from build123d import *

# Parameters (mm, degrees)
SKETCH1_R           = 0.5
SKETCH1_R_2         = 1.375
BOSS_EXTRUDE1_DEPTH = 2
SKETCH4_R           = 4.5
SKETCH4_R_2         = 2.5
BOSS_EXTRUDE3_DEPTH = 3
CUT_EXTRUDE3_START  = -3
CUT_EXTRUDE3_DEPTH  = 3
SKETCH6_W           = 34.029642768
SKETCH6_H           = 33.796563024
CUT_EXTRUDE4_DEPTH  = 22.43595111
SKETCH7_W           = 10.1
SKETCH7_H           = 10.1
BOSS_EXTRUDE4_DEPTH = 1.25
SKETCH8_W           = 1.25
SKETCH8_H           = 10.1
BOSS_EXTRUDE5_DEPTH = 2


with BuildPart() as part:
    # Sketch1 → Boss-Extrude1 (new body)
    with BuildSketch(Plane(origin=(0, 0, 0), x_dir=(1, 0, 0), z_dir=(0, 1, 0))):
        with BuildLine():
            Line((-4, 4), (-2.467435953, 13.402193757))
            ThreePointArc((-2.467435953, 13.402193757), (0, 15.5), (2.467435953, 13.402193757))
            Line((2.467435953, 13.402193757), (4, 4))
            Line((4, 4), (12.448472752, 2.459445505))
            ThreePointArc((12.448472752, 2.459445505), (14.5, 0), (12.448472752, -2.459445505))
            Line((12.448472752, -2.459445505), (4, -4))
            Line((4, -4), (2.467435953, -13.402193757))
            ThreePointArc((2.467435953, -13.402193757), (0, -15.5), (-2.467435953, -13.402193757))
            Line((-2.467435953, -13.402193757), (-4, -4))
            Line((-4, -4), (-12.448472752, -2.459445505))
            ThreePointArc((-12.448472752, -2.459445505), (-14.5, 0), (-12.448472752, 2.459445505))
            Line((-12.448472752, 2.459445505), (-4, 4))
        make_face()
        with Locations(Location((0, 12, 0), (0, 0, 270))):
            Circle(SKETCH1_R, mode=Mode.SUBTRACT)
        with Locations(Location((0, 9.5, 0), (0, 0, 270))):
            Circle(SKETCH1_R, mode=Mode.SUBTRACT)
        with Locations(Location((0, 7.5, 0), (0, 0, 270))):
            Circle(SKETCH1_R, mode=Mode.SUBTRACT)
        with Locations(Location((12, 0, 0), (0, 0, 270))):
            Circle(SKETCH1_R, mode=Mode.SUBTRACT)
        with Locations(Location((9.5, 0, 0), (0, 0, 270))):
            Circle(SKETCH1_R, mode=Mode.SUBTRACT)
        with Locations(Location((7.5, 0, 0), (0, 0, 270))):
            Circle(SKETCH1_R, mode=Mode.SUBTRACT)
        with Locations(Location((0, -12, 0), (0, 0, 270))):
            Circle(SKETCH1_R, mode=Mode.SUBTRACT)
        with Locations(Location((0, -9.5, 0), (0, 0, 270))):
            Circle(SKETCH1_R, mode=Mode.SUBTRACT)
        with Locations(Location((0, -7.5, 0), (0, 0, 270))):
            Circle(SKETCH1_R, mode=Mode.SUBTRACT)
        with Locations(Location((-12, 0, 0), (0, 0, 270))):
            Circle(SKETCH1_R, mode=Mode.SUBTRACT)
        with Locations(Location((-9.5, 0, 0), (0, 0, 270))):
            Circle(SKETCH1_R, mode=Mode.SUBTRACT)
        with Locations(Location((-7.5, 0, 0), (0, 0, 270))):
            Circle(SKETCH1_R, mode=Mode.SUBTRACT)
        with Locations(Location((0, 0, 0), (0, 0, 270))):
            Circle(SKETCH1_R_2, mode=Mode.SUBTRACT)
    extrude(amount=BOSS_EXTRUDE1_DEPTH)

    # Sketch4 → Boss-Extrude3 (add)
    with BuildSketch(Plane.XZ):
        with Locations(Location((0, 0, 0), (0, 0, 90))):
            Circle(SKETCH4_R)
        with Locations(Location((0, 0, 0), (0, 0, 270))):
            Circle(SKETCH4_R_2, mode=Mode.SUBTRACT)
    extrude(amount=BOSS_EXTRUDE3_DEPTH)

    # Sketch5 → Cut-Extrude3 (cut)
    with BuildSketch(Plane.XZ.offset(3).offset(CUT_EXTRUDE3_START)):
        with BuildLine():
            Line((0.299038106, 2.482050808), (0, 3))
            Line((0, 3), (-0.299038106, 2.482050808))
            ThreePointArc((-0.299038106, 2.482050808), (-0.391086163, 2.469220851), (-0.482593741, 2.452978451))
            Line((-0.482593741, 2.452978451), (-0.927050983, 2.853169549))
            Line((-0.927050983, 2.853169549), (-1.051398019, 2.268162738))
            ThreePointArc((-1.051398019, 2.268162738), (-1.134976249, 2.22751631), (-1.216985951, 2.183791473))
            Line((-1.216985951, 2.183791473), (-1.763355757, 2.427050983))
            Line((-1.763355757, 2.427050983), (-1.70083977, 1.832251096))
            ThreePointArc((-1.70083977, 1.832251096), (-1.767766953, 1.767766953), (-1.832251096, 1.70083977))
            Line((-1.832251096, 1.70083977), (-2.427050983, 1.763355757))
            Line((-2.427050983, 1.763355757), (-2.183791473, 1.216985951))
            ThreePointArc((-2.183791473, 1.216985951), (-2.22751631, 1.134976249), (-2.268162738, 1.051398019))
            Line((-2.268162738, 1.051398019), (-2.853169549, 0.927050983))
            Line((-2.853169549, 0.927050983), (-2.452978451, 0.482593741))
            ThreePointArc((-2.452978451, 0.482593741), (-2.469220851, 0.391086163), (-2.482050808, 0.299038106))
            Line((-2.482050808, 0.299038106), (-3, 0))
            Line((-3, 0), (-2.482050808, -0.299038106))
            ThreePointArc((-2.482050808, -0.299038106), (-2.469220851, -0.391086163), (-2.452978451, -0.482593741))
            Line((-2.452978451, -0.482593741), (-2.853169549, -0.927050983))
            Line((-2.853169549, -0.927050983), (-2.268162738, -1.051398019))
            ThreePointArc((-2.268162738, -1.051398019), (-2.22751631, -1.134976249), (-2.183791473, -1.216985951))
            Line((-2.183791473, -1.216985951), (-2.427050983, -1.763355757))
            Line((-2.427050983, -1.763355757), (-1.832251096, -1.70083977))
            ThreePointArc((-1.832251096, -1.70083977), (-1.767766953, -1.767766953), (-1.70083977, -1.832251096))
            Line((-1.70083977, -1.832251096), (-1.763355757, -2.427050983))
            Line((-1.763355757, -2.427050983), (-1.216985951, -2.183791473))
            ThreePointArc((-1.216985951, -2.183791473), (-1.134976249, -2.22751631), (-1.051398019, -2.268162738))
            Line((-1.051398019, -2.268162738), (-0.927050983, -2.853169549))
            Line((-0.927050983, -2.853169549), (-0.482593741, -2.452978451))
            ThreePointArc((-0.482593741, -2.452978451), (-0.391086163, -2.469220851), (-0.299038106, -2.482050808))
            Line((-0.299038106, -2.482050808), (0, -3))
            Line((0, -3), (0.299038106, -2.482050808))
            ThreePointArc((0.299038106, -2.482050808), (0.391086163, -2.469220851), (0.482593741, -2.452978451))
            Line((0.482593741, -2.452978451), (0.927050983, -2.853169549))
            Line((0.927050983, -2.853169549), (1.051398019, -2.268162738))
            ThreePointArc((1.051398019, -2.268162738), (1.134976249, -2.22751631), (1.216985951, -2.183791473))
            Line((1.216985951, -2.183791473), (1.763355757, -2.427050983))
            Line((1.763355757, -2.427050983), (1.70083977, -1.832251096))
            ThreePointArc((1.70083977, -1.832251096), (1.767766953, -1.767766953), (1.832251096, -1.70083977))
            Line((1.832251096, -1.70083977), (2.427050983, -1.763355757))
            Line((2.427050983, -1.763355757), (2.183791473, -1.216985951))
            ThreePointArc((2.183791473, -1.216985951), (2.22751631, -1.134976249), (2.268162738, -1.051398019))
            Line((2.268162738, -1.051398019), (2.853169549, -0.927050983))
            Line((2.853169549, -0.927050983), (2.452978451, -0.482593741))
            ThreePointArc((2.452978451, -0.482593741), (2.469220851, -0.391086163), (2.482050808, -0.299038106))
            Line((2.482050808, -0.299038106), (3, 0))
            Line((3, 0), (2.482050808, 0.299038106))
            ThreePointArc((2.482050808, 0.299038106), (2.469220851, 0.391086163), (2.452978451, 0.482593741))
            Line((2.452978451, 0.482593741), (2.853169549, 0.927050983))
            Line((2.853169549, 0.927050983), (2.268162738, 1.051398019))
            ThreePointArc((2.268162738, 1.051398019), (2.22751631, 1.134976249), (2.183791473, 1.216985951))
            Line((2.183791473, 1.216985951), (2.427050983, 1.763355757))
            Line((2.427050983, 1.763355757), (1.832251096, 1.70083977))
            ThreePointArc((1.832251096, 1.70083977), (1.767766953, 1.767766953), (1.70083977, 1.832251096))
            Line((1.70083977, 1.832251096), (1.763355757, 2.427050983))
            Line((1.763355757, 2.427050983), (1.216985951, 2.183791473))
            ThreePointArc((1.216985951, 2.183791473), (1.134976249, 2.22751631), (1.051398019, 2.268162738))
            Line((1.051398019, 2.268162738), (0.927050983, 2.853169549))
            Line((0.927050983, 2.853169549), (0.482593741, 2.452978451))
            ThreePointArc((0.482593741, 2.452978451), (0.391086163, 2.469220851), (0.299038106, 2.482050808))
        make_face()
    extrude(amount=CUT_EXTRUDE3_DEPTH, mode=Mode.SUBTRACT)

    # Sketch6 → Cut-Extrude4 (cut, through all)
    with BuildSketch(Plane(origin=(0, 0, 0), x_dir=(-1, 0, 0), z_dir=(0, -1, 0))):
        Rectangle(SKETCH6_W, SKETCH6_H)
    extrude(amount=-CUT_EXTRUDE4_DEPTH, mode=Mode.SUBTRACT)

    # Sketch7 → Boss-Extrude4 (add)
    with BuildSketch(Plane(origin=(0, 0, 0), x_dir=(1, 0, 0), z_dir=(0, 1, 0))):
        Rectangle(SKETCH7_W, SKETCH7_H)
    extrude(amount=BOSS_EXTRUDE4_DEPTH)

    # Sketch8 → Boss-Extrude5 (add)
    with BuildSketch(Plane(origin=(0, 1.25, 0), x_dir=(1, 0, 0), z_dir=(0, 1, 0))):
        with Locations((-4.425, 0)):
            Rectangle(SKETCH8_W, SKETCH8_H)
        with Locations((4.425, 0)):
            Rectangle(SKETCH8_W, SKETCH8_H)
    extrude(amount=BOSS_EXTRUDE5_DEPTH)


solid = part.part
For this review, take the finished solid that the model builds, in its own axes (mm). A direction names the side the tool comes from. Round coordinates to 2 decimals unless told otherwise and drop trailing zeros. Loops run counter-clockwise (first coordinate to the right, second up) from the corner with the lowest first, then second, coordinate; pieces in that order, holes last. Notation, with made-up numbers: (7, 68) - (47, 68) arc R24 ccw to (47, 90) - close; hole circle Ø2 at (-31, 63.25). An arc over 180 degrees is marked (long way). Use one line per item in the form item = value.
1) We need section C-C on x = 2. Write out the cut boundary in (y, z), then the cut area to 3 significant figures.
Solutions:
outline = (-3, -4.03) - (0, -4.03) - (0, -5.05) - (1.25, -5.05) - (1.25, 5.05) - (0, 5.05) - (0, 4.03) - (-3, 4.03) - (-3, 1.72) - (0, 1.72) - (0, -1.72) - (-3, -1.72) - close
area = 26.5 mm2
2) Clearance check with flat-ended pins moving along their axes: P1, Ø2.5, axis at x = -1.5, z = 1.5, coming from the +Y side; P2, Ø1.8, axis at x = -1.5, z = 0, coming from the -Y side; P3, Ø1, axis at x = -2.5, y = -2, coming from the +Z side. State where each tip first meets the part, or that it passes through.
Solutions:
P1 = 1.25
P2 = 0
P3 = 4.03
3) Wall thickness on probe 1 along X at (y, z) = (2.75, -0.5); probe 2 along Y at (x, z) = (3, -3.75); probe 3 along Y at (x, z) = (4.25, 4): over which ranges is each line inside the solid? List them lowest first.
Solutions:
probe_1 = -5.05 to -3.8, 3.8 to 5.05
probe_2 = 0 to 1.25
probe_3 = 0 to 3.25
4) We need section B-B on x = -4. Write out the cut boundary in (y, z), then the cut area to 3 significant figures.
Solutions:
outline = (-3, -2.06) - (0, -2.06) - (0, -5.05) - (3.25, -5.05) - (3.25, 5.05) - (0, 5.05) - (0, 2.06) - (-3, 2.06) - close
area = 45.2 mm2
5) Mouldability with a two-part tool opening along Z and no side actions: class faces 1 (the face through (0, 1.25, 0)), 2 (the face through (0, 0, 0)), 3 (the face through (-1.352, -1.479, 4.292)) as pulls with the +Z half, pulls with the -Z half, needs draft (parallel to the pull), parting line crosses it, or undercut.
Solutions:
face_1 = needs draft
face_2 = undercut
face_3 = parting line crosses it
6) We need section A-A on y = 2.5. Write out the cut boundary in (x, z).
Solutions:
outline = (-5.05, -5.05) - (-3.8, -5.05) - (-3.8, 5.05) - (-5.05, 5.05) - close; (3.8, -5.05) - (5.05, -5.05) - (5.05, 5.05) - (3.8, 5.05) - close
7) Tool access review of faces 4 (the face through (-5.05, 2, 0)), 5 (the face through (-3.8, 2, 0)), 6 (the face through (-4.6, 0, -1.2)): name each direction out of +Z, -Z, +X, -X, +Y, -Y from which nothing blocks a thin tool from reaching the whole face with its end or side.
Solutions:
face_4 = +Z, -Z, -X, +Y, -Y
face_5 = +Z, -Z, +Y
face_6 = -Y
